```python
from build123d import *

# Parameters (mm, degrees)
SKETCH_1_W          = 10
SKETCH_1_H          = 15
EXTRUDE_1_DEPTH     = 20
FILLET_1_RADIUS     = 5
FILLET_1_LENGTH     = 20
SKETCH_2_R          = 2.5
EXTRUDE_2_DEPTH     = 10
SKETCH_3_R          = 2.5
CUT_EXTRUDE_1_DEPTH = 28.041634566
SKETCH_4_R          = 1.5
EXTRUDE_3_DEPTH     = 100


with BuildPart() as part:
    # 스케치1 → 보스-돌출1 (new body)
    with BuildSketch(Plane(origin=(0, 0, 0), x_dir=(0, 0, -1), z_dir=(1, 0, 0))):
        Rectangle(SKETCH_1_W, SKETCH_1_H)
    extrude(amount=EXTRUDE_1_DEPTH)

    # 필렛1: full round fillet: the end face becomes a half cylinder, R = half its width
    fillet_1_face = Plane((10, -7.5, 0), x_dir=(1, 0, 0), z_dir=(0, -1, 0))  # on the end face: x along it, z out of the body
    fillet_1_slab = fillet_1_face.offset(-FILLET_1_RADIUS / 2) * Box(FILLET_1_LENGTH, 2 * FILLET_1_RADIUS, FILLET_1_RADIUS, mode=Mode.PRIVATE)  # the body's end, R deep
    fillet_1_round = Plane((10, -2.5, 0), x_dir=(0, -1, 0), z_dir=(1, 0, 0)) * Cylinder(FILLET_1_RADIUS, FILLET_1_LENGTH, mode=Mode.PRIVATE)  # its axis R under the face
    add(fillet_1_slab - fillet_1_round, mode=Mode.SUBTRACT)

    # 스케치2 → 보스-돌출2 (add)
    with BuildSketch(Plane(origin=(0, 7.5, 0), x_dir=(1, 0, 0), z_dir=(0, 1, 0))):
        with Locations(Location((5, 0, 0), (0, 0, 90))):
            Circle(SKETCH_2_R)
    extrude(amount=EXTRUDE_2_DEPTH)

    # 스케치3 → 컷-돌출1 (cut, through all)
    with BuildSketch(Plane(origin=(20, 0, 0), x_dir=(0, 0, -1), z_dir=(1, 0, 0))):
        with Locations((0, -2.5)):
            Circle(SKETCH_3_R)
    extrude(amount=-CUT_EXTRUDE_1_DEPTH, mode=Mode.SUBTRACT)

    # 스케치4 → 보스-돌출3 (add)
    with BuildSketch(Plane(origin=(20, 0, 0), x_dir=(0, 0, -1), z_dir=(1, 0, 0))):
        with Locations((0, 5.5)):
            Circle(SKETCH_4_R)
    extrude(amount=EXTRUDE_3_DEPTH)


solid = part.part
```
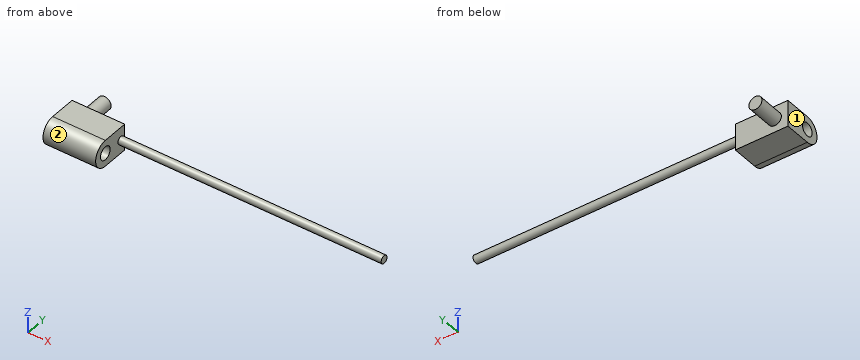
CAD build for the part. Positions are in the model's coordinates, mm. Face numbers are marked on the shaded views. Coordinates: 2 decimals unless noted, no trailing zeros. Write each loop counter-clockwise with the first axis right and the second up, starting at its lowest first coordinate (ties: lowest second). Pieces come first, ordered by that corner, then holes.
(1) Cut at A-A, the plane z = 0. List the corners of the cut face in (x, y), and give its area (3 significant figures).
(2) Drill centre lines: probe 1 along Y at (x, z) = (14.25, 0); probe 2 along X at (y, z) = (4.25, 1); probe 3 along X at (y, z) = (12.5, 0). Where is each one in solid material? Low to high.
(3) Cut at C-C, the plane x = 18.5. List the corners of the cut face in (y, z), and give its area (3 significant figures).
(4) Cut at B-B, the plane y = 5.5. List the corners of the cut face in (x, z).
(5) Cut at D-D, the plane x = 112.5. List the corners of the cut face in (y, z).
(6) Two-plate mould, pull along X, no slides. Class the marked faces 1 and 2: +X half, -X half, draft (parallel to the pull), parting line (faces both ways), or undercut.
(7) Flat gauge pins, fed straight in: pin 1 (3 mm diameter, centred on x = 40, z = -2.5, fed in from -Y); pin 2 (12 mm diameter, centred on x = 56, y = 2.5, fed in from -Z); pin 3 (6 mm diameter, centred on x = 83.5, y = 9.5, fed in from +Z); pin 4 (4 mm diameter, centred on x = 52, y = 1.5, fed in from +Z). Where does each tip first touch, or does it go through?
Geometry says:
1. outline: (0, -7.5) - (20, -7.5) - (20, -5) - (0, -5) - close; (0, 0) - (20, 0) - (20, 4) - (120, 4) - (120, 7) - (20, 7) - (20, 7.5) - (7.5, 7.5) - (7.5, 17.5) - (2.5, 17.5) - (2.5, 7.5) - (0, 7.5) - close
1. area: 550 mm2
2. probe 1: y = -7.5 to -5, 0 to 7.5
2. probe 2: x = 0 to 20
2. probe 3: x = 2.5 to 7.5
3. outline: (-2.5, -5) - (7.5, -5) - (7.5, 5) - (-2.5, 5) arc R5 ccw to start; hole circle Ø5 at (-2.5, 0)
3. area: 120 mm2
4. outline: (0, -5) - (20, -5) - (20, -1.5) - (120, -1.5) - (120, 1.5) - (20, 1.5) - (20, 5) - (0, 5) - close
5. outline: circle Ø3 at (5.5, 0)
6. face 1: -X half
6. face 2: draft
7. pin 1: stops at y = 4.38
7. pin 2: stops at z = -1.5
7. pin 3: stops at z = 1.12
7. pin 4: passes through
